from build123d import *

# Parameters (mm, degrees)
CROQUIS1_R              = 50
SALIENTE_EXTRUIR1_DEPTH = 50
CROQUIS2_R              = 25
SALIENTE_EXTRUIR2_DEPTH = 500
CROQUIS3_R              = 50
SALIENTE_EXTRUIR3_DEPTH = 100
CORTAR_EXTRUIR1_START   = -50
CROQUIS4_R              = 25
CORTAR_EXTRUIR1_DEPTH   = 50


with BuildPart() as part:
    # Croquis1 → Saliente-Extruir1 (new, symmetric)
    with BuildSketch(Plane(origin=(0, 0, 0), x_dir=(0, 0, -1), z_dir=(1, 0, 0))):
        Circle(CROQUIS1_R)
    extrude(amount=SALIENTE_EXTRUIR1_DEPTH, both=True)

    # Croquis2 → Saliente-Extruir2 (add)
    with BuildSketch(Plane(origin=(0, 0, 0), x_dir=(1, 0, 0), z_dir=(0, 1, 0))):
        with Locations(Location((0, 0, 0), (0, 0, 90))):
            Circle(CROQUIS2_R)
    extrude(amount=SALIENTE_EXTRUIR2_DEPTH)

    # Croquis3 → Saliente-Extruir3 (add)
    with BuildSketch(Plane(origin=(0, 500, 0), x_dir=(1, 0, 0), z_dir=(0, 1, 0))):
        with Locations(Location((0, 0, 0), (0, 0, 270))):
            Circle(CROQUIS3_R)
    extrude(amount=SALIENTE_EXTRUIR3_DEPTH)

    # Croquis4 → Cortar-Extruir1 (cut)
    with BuildSketch(Plane(origin=(0, 600, 0), x_dir=(1, 0, 0), z_dir=(0, 1, 0)).offset(CORTAR_EXTRUIR1_START)):
        with Locations(Location((0, 0, 0), (0, 0, 90))):
            Circle(CROQUIS4_R)
    extrude(amount=CORTAR_EXTRUIR1_DEPTH, mode=Mode.SUBTRACT)


solid = part.part
The listing builds one solid part. Answer for the finished solid, in the listing's coordinates (mm). A direction names the side the tool comes from. Coordinates: 2 decimals unless noted, no trailing zeros. Order: outer loops, then holes, each group sorted by start corner. A loop starts at its lowest first (then second) coordinate and runs counter-clockwise, first axis right, second up.
Q1. A cutting plane is placed at A-A, the plane z = 40. Write down the section's boundary in (x, y), and give its area (3 significant figures).
Q2. A cutting plane is placed at C-C, the plane z = 0. Write down the section's boundary in (x, y), and give its area (3 significant figures).
Q3. Given P1, Ø2, axis at y = 127.5, z = 22, coming from the +X side; P2, Ø3, axis at x = -20.5, y = 303.5, coming from the +Z side; P3, Ø1, axis at x = 3.5, y = 356.5, coming from the +Z side, each flat-ended and moving along its own axis, determine where each tip first touches the part or whether it passes through.
Q4. For a pull along Z with two mould halves and no side action, classify faces 1 (the face through (-50, 1, 1)), 2 (the face through (-7.509, 268.454, -23.846)), 3 (the face through (0, 550, 0)) as pulls with the +Z half, pulls with the -Z half, needs draft (parallel to the pull), parting line crosses it, or undercut.
Q5. A cutting plane is placed at B-B, the plane x = 0. Write down the section's boundary in (y, z), and give its area (3 significant figures).
Q6. Consider line 1 (X direction, y = 587, z = 0); line 2 (Y direction, x = -33, z = 4.5); line 3 (Y direction, x = 16.5, z = 20). Determine where each line is inside the solid, lowest interval first.
Q7. A cutting plane is placed at D-D, the plane x = 43. Write down the section's boundary in (y, z), and give its area (3 significant figures).
Q8. Which of the six approach directions +Z, -Z, +X, -X, +Y, -Y give full straight-line access (tool end or side, diameter ignored) to faces 4 (the face through (15.02, 549.3, 47.69)), 5 (the face through (50, 1, 1)), 6 (the face through (22.9, 500, 10.4))?
Answers follow:
1. outline: (-50, -30) - (50, -30) - (50, 30) - (-50, 30) - close; (-30, 500) - (30, 500) - (30, 600) - (-30, 600) - close
1. area: 12,000 mm2
2. outline: (-50, -50) - (50, -50) - (50, 50) - (25, 50) - (25, 500) - (50, 500) - (50, 600) - (25, 600) - (25, 550) - (-25, 550) - (-25, 600) - (-50, 600) - (-50, 500) - (-25, 500) - (-25, 50) - (-50, 50) - close
2. area: 40,000 mm2
3. P1: stops at x = 13.56
3. P2: stops at z = 16.25
3. P3: stops at z = 24.82
4. face 1: needs draft
4. face 2: parting line crosses it
4. face 3: undercut
5. outline: (43.3, -25) - (500, -25) - (500, -50) - (600, -50) - (600, -25) - (550, -25) - (550, 25) - (600, 25) - (600, 50) - (500, 50) - (500, 25) - (43.3, 25) arc R50 ccw (long way) to start
5. area: 38,000 mm2
6. line 1: x = -50 to -25, 25 to 50
6. line 2: y = -49.8 to 49.8, 500 to 600
6. line 3: y = -45.83 to 45.83, 500 to 600
7. outline: circle Ø100 at (0, 0); (500, -25.51) - (600, -25.51) - (600, 25.51) - (500, 25.51) - close
7. area: 13,000 mm2
8. face 4: +Y
8. face 5: +Z, -Z, +X, +Y, -Y
8. face 6: none
